CAD build for the part. Positions are in the model's coordinates, mm. Coordinates: 2 decimals unless noted, no trailing zeros. Loops run counter-clockwise (first coordinate to the right, second up) from the corner with the lowest first, then second, coordinate; pieces in that order, holes last. Notation, with made-up numbers: (-33, 9.25) -> (-28, 9.25) arc R36 ccw to (-28, 45.25) -> close; hole circle Ø5 at (20, 31.25). An arc over 180 degrees is marked (long way). Answer as a JSON object with one key per item and string values. Group by question number.
from build123d import *

# Parameters (mm, degrees)
SKETCH1_W           = 16.0528
SKETCH1_H           = 0.1524
BOSS_EXTRUDE1_DEPTH = 609.6
SKETCH2_R           = 2.54
CUT_EXTRUDE1_DEPTH  = 508


with BuildPart() as part:
    # Sketch1 → Boss-Extrude1 (new body)
    with BuildSketch(Plane(origin=(0, 0, 0), x_dir=(1, 0, 0), z_dir=(0, 1, 0))):
        Polygon((32.512, 7.0612), (32.512, 8.4582), (40.005, 8.4582), (40.005, 0), (0, 0), (0, 8.4582), (7.493, 8.4582), (7.493, 7.0612), (2.032, 7.0612), (2.032, 2.54), (37.973, 2.54), (37.973, 7.0612), align=None)
        Polygon((13.7541, 5.269994695), (13.7541, 2.54), (26.2509, 2.54), (26.2509, 5.269994695), (25.298905305, 4.318), (14.706094695, 4.318), align=None)
        with Locations((20.0025, -0.0762)):
            Rectangle(SKETCH1_W, SKETCH1_H)
    extrude(amount=BOSS_EXTRUDE1_DEPTH)

    # Sketch2 → Cut-Extrude1 (cut)
    with BuildSketch(Plane(origin=(0, 0, -4.318), x_dir=(-1, 0, 0), z_dir=(0, 0, -1))):
        with Locations((-20.0025, 574.675)):
            Circle(SKETCH2_R)
        with Locations((-20.0025, 514.731)):
            Circle(SKETCH2_R)
        with Locations((-20.0025, 454.787)):
            Circle(SKETCH2_R)
        with Locations((-20.0025, 394.843)):
            Circle(SKETCH2_R)
        with Locations((-20.0025, 334.899)):
            Circle(SKETCH2_R)
        with Locations((-20.0025, 274.955)):
            Circle(SKETCH2_R)
        with Locations((-20.0025, 215.011)):
            Circle(SKETCH2_R)
        with Locations((-20.0025, 155.067)):
            Circle(SKETCH2_R)
        with Locations((-20.0025, 95.123)):
            Circle(SKETCH2_R)
        with Locations((-20.0025, 35.179)):
            Circle(SKETCH2_R)
    extrude(amount=-CUT_EXTRUDE1_DEPTH, mode=Mode.SUBTRACT)


solid = part.part
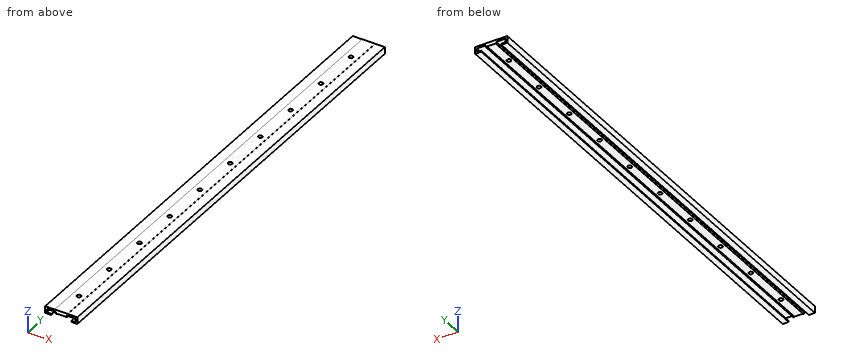
Item 1: Drill centre lines: L1, parallel to X at y = 338.5, z = -3 (3 decimals); L2, parallel to X at y = 168.5, z = -7.75 (3 decimals); L3, parallel to X at y = 422, z = -7 (3 decimals). Where is each one in solid material? Low to high.
Item 2: Band-saw the part on A-A, the plane y = 318. List the corners of the cut face in (x, z) (3 decimals).
Item 3: Flat gauge pins, fed straight in: P1, Ø4.5, axis at x = 20, y = 514.73, coming from the -Z side; P2, Ø1.1, axis at y = 349, z = -8, coming from the -X side; P3, Ø6.5, axis at x = 20, y = 215.01, coming from the -Z side; P4, Ø6, axis at x = 35, y = 384.5, coming from the +Z side. Where does each tip first touch, or does it go through?
Reply:
{
 "1": {"L1": "0 to 2.032, 13.754 to 26.251, 37.973 to 40.005", "L2": "0 to 7.493, 32.512 to 40.005", "L3": "0 to 2.032, 37.973 to 40.005"},
 "2": {"outline": "(0, -8.458) -> (7.493, -8.458) -> (7.493, -7.061) -> (2.032, -7.061) -> (2.032, -2.54) -> (13.754, -2.54) -> (13.754, -5.27) -> (14.706, -4.318) -> (25.299, -4.318) -> (26.251, -5.27) -> (26.251, -2.54) -> (37.973, -2.54) -> (37.973, -7.061) -> (32.512, -7.061) -> (32.512, -8.458) -> (40.005, -8.458) -> (40.005, 0) -> (28.029, 0) -> (28.029, 0.152) -> (11.976, 0.152) -> (11.976, 0) -> (0, 0) -> close"},
 "3": {"P1": "through", "P2": "x = 0", "P3": "z = -4.32", "P4": "z = 0"}
}
